CAD build for the part. Positions are in the model's coordinates, mm. Face numbers are marked on the shaded views. A direction names the side the tool comes from. Coordinates: 2 decimals unless noted, no trailing zeros. Write each loop counter-clockwise with the first axis right and the second up, starting at its lowest first coordinate (ties: lowest second). Pieces come first, ordered by that corner, then holes. Notation, with made-up numbers: M -29.5,12 L 4.5,12 A20 ccw 4.5,19 Z; hole C 23,-3 d4. An arc over 180 degrees is marked long. Put each result on its own line as item: value. Start each with the question number.
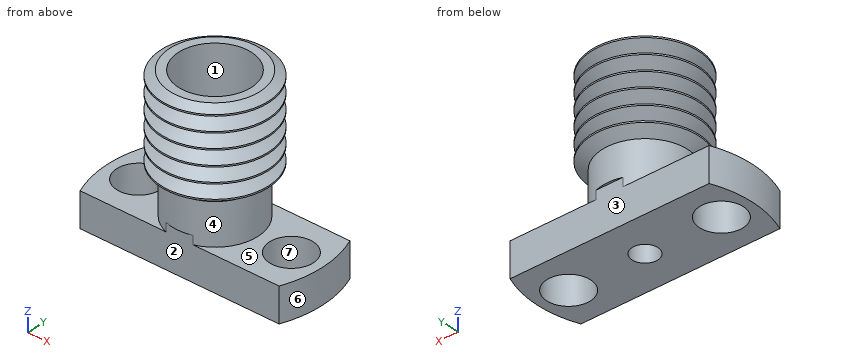
```python
from build123d import *

# Parameters (mm, degrees)
SKETCH5_OUTSIDE_W   = 23.578
SKETCH5_OUTSIDE_H   = 23.578
SKETCH5_OUTSIDE_R   = 1.2954
CE_00_500_355_DEPTH = 2.54
LPATTERN4_COUNT     = 6
LPATTERN4_PITCH     = 0.907142857


with BuildPart() as part:
    # Sketch1 → Revolve1 (revolve)
    with BuildSketch(Plane(origin=(0, 0, 0), x_dir=(0, 0, -1), z_dir=(1, 0, 0)), mode=Mode.PRIVATE) as revolve1_sk:
        Polygon((-2.032, 2.54), (-4.512366142, 2.54), (-4.878983563, 3.175), (-9.553072205, 3.175), (-9.846366142, 2.667), (-9.846366142, 2.159), (-6.793879368, 2.159), (-6.793879368, 1.524), (-3.100370371, 1.524), (-3.100370371, 0.762), (0, 0.762), (0, 8.255), (-2.032, 8.255), align=None)
    revolve(revolve1_sk.sketch.rotate(Axis((0, 0, 6.793879368), (0, 0, -1)), 90), axis=Axis((0, 0, 6.793879368), (0, 0, -1)))

    # Sketch5 outside → CE-00 500 355 (cut)
    # profile 1 of 3: a face of its own
    with BuildSketch(Plane.XY):
        Rectangle(SKETCH5_OUTSIDE_W, SKETCH5_OUTSIDE_H)
        with BuildLine():
            Line((5.873664189, -2.413), (-5.873664189, -2.413))
            ThreePointArc((-5.873664189, -2.413), (-6.35, 0), (-5.873664189, 2.413))
            Line((-5.873664189, 2.413), (5.873664189, 2.413))
            ThreePointArc((5.873664189, 2.413), (6.35, 0), (5.873664189, -2.413))
        make_face(mode=Mode.SUBTRACT)
    # profile 2 of 3: a face of its own
    with BuildSketch(Plane.XY):
        with Locations(Location((-4.5085, 0, 0), (0, 0, 180))):
            Circle(SKETCH5_OUTSIDE_R)
    # profile 3 of 3: a face of its own
    with BuildSketch(Plane.XY):
        with Locations(Location((4.5085, 0, 0), (0, 0, 180))):
            Circle(SKETCH5_OUTSIDE_R)
    extrude(amount=CE_00_500_355_DEPTH, mode=Mode.SUBTRACT)

    # Sketch4 → Cut-Revolve1 (revolve, cut)
    with BuildSketch(Plane(origin=(0, 0, 0), x_dir=(0, 0, -1), z_dir=(1, 0, 0)), mode=Mode.PRIVATE) as cut_revolve1_sk:
        Polygon((-9.523742812, 3.2766), (-9.055506686, 2.465591241), (-8.587270561, 3.2766), align=None)
    cut_revolve1 = revolve(cut_revolve1_sk.sketch.rotate(Axis((0, 0, -0.492318307), (0, 0, 1)), 270), axis=Axis((0, 0, -0.492318307), (0, 0, 1)), mode=Mode.SUBTRACT)

    # LPattern4: Cut-Revolve1 ×6
    with Locations(*[(0, 0, -i * LPATTERN4_PITCH) for i in range(1, LPATTERN4_COUNT)]):
        add(cut_revolve1, mode=Mode.SUBTRACT)


solid = part.part
```
(1) Slice it at B-B, the plane x = -4. Write the cut outline in (y, z).
(2) Drop flat-ended pins along their axis: pin 1 (3 mm diameter, centred on x = 0.5, z = 3, fed in from +Y); pin 2 (1 mm diameter, centred on x = 0.5, z = 3, fed in from -Y); pin 3 (2 mm diameter, centred on x = -2, z = 2, fed in from -Y); pin 4 (3 mm diameter, centred on x = -2.5, y = 2, fed in from -Z). Give the stop position or say it passes through.
(3) Slice it at D-D, the plane x = 5.5. Write the cut outline in (y, z).
(4) Slice it at A-A, the plane z = 1.75. Write the cut outline in (x, y), then the cut area to 3 significant figures.
(5) Which spindle directions (+Z, -Z, +X, -X, +Y, -Y) get a long thin tool onto all of the face, cutting with end or side? Do the marked faces 1, 2, 3 and 4. Say none if no direction does.
(6) Two-plate mould, pull along Y, no slides. Class the marked faces 5, 6 and 7: +Y half, -Y half, draft (parallel to the pull), parting line (faces both ways), or undercut.
(7) Slice it at C-C, the plane z = 7.5. Write the cut outline in (x, y).
(8) Drill centre lines: line 1 (X direction, y = 0.5, z = 1); line 2 (Z direction, x = -1.75, y = 2.5); line 3 (Y direction, x = 0, z = 1.8). Where is each one in solid material? Low to high. Write a range as [from, to].
Result set:
1. outline: M -2.41,0 L -1.19,0 L -1.19,2.03 L -2.41,2.03 Z; M 1.19,0 L 2.41,0 L 2.41,2.03 L 1.19,2.03 Z
2. pin 1: stops at y = 2.54
2. pin 2: stops at y = -2.54
2. pin 3: stops at y = -2.41
2. pin 4: stops at z = 0
3. outline: M -2.41,0 L -0.83,0 L -0.83,2.03 L -2.41,2.03 Z; M 0.83,0 L 2.41,0 L 2.41,2.03 L 0.83,2.03 Z
4. outline: M -5.87,-2.41 L 5.87,-2.41 A6.35 ccw 5.87,2.41 L -5.87,2.41 A6.35 ccw Z; hole C -4.51,0 d2.59; hole C 0,0 d1.52; hole C 4.51,0 d2.59
4. area: 47.4 mm^2
5. face 1: +Z
5. face 2: -Z, +X, -X, -Y
5. face 3: -Z, +X, -X, +Y
5. face 4: none
6. face 5: draft
6. face 6: parting line
6. face 7: undercut
7. outline: C 0,0 d5.83; hole C 0,0 d4.32
8. line 1: x = [-6.33, -5.7], [-3.31, -0.58], [0.58, 3.31], [5.7, 6.33]
8. line 2: z = [4.86, 5.09], [5.77, 6], [6.67, 6.9], [7.58, 7.81], [8.49, 8.72], [9.39, 9.62]
8. line 3: y = [-2.41, -0.76], [0.76, 2.41]
